from build123d import *

# Parameters (mm, degrees)
SKETCH1_R           = 7.5
BOSS_EXTRUDE1_DEPTH = 8
SKETCH2_R           = 7.5
BOSS_EXTRUDE2_DEPTH = 2
SKETCH3_R           = 4
BOSS_EXTRUDE3_DEPTH = 20
SKETCH4_R           = 5
BOSS_EXTRUDE4_DEPTH = 15


with BuildPart() as part:
    # Sketch1 → Boss-Extrude1 (new body)
    with BuildSketch(Plane(origin=(0, 0, 0), x_dir=(1, 0, 0), z_dir=(0, 1, 0))):
        Circle(SKETCH1_R)
        Polygon((5.773502692, 0), (2.886751346, 5), (-2.886751346, 5), (-5.773502692, 0), (-2.886751346, -5), (2.886751346, -5), align=None, mode=Mode.SUBTRACT)
    extrude(amount=BOSS_EXTRUDE1_DEPTH)

    # Sketch2 → Boss-Extrude2 (add)
    with BuildSketch(Plane.XZ):
        Circle(SKETCH2_R)
    extrude(amount=BOSS_EXTRUDE2_DEPTH)

    # Sketch3 → Boss-Extrude3 (add)
    with BuildSketch(Plane.XZ.offset(2)):
        Circle(SKETCH3_R)
    extrude(amount=BOSS_EXTRUDE3_DEPTH)

    # Sketch4 → Boss-Extrude4 (add)
    with BuildSketch(Plane.XZ.offset(22)):
        Circle(SKETCH4_R)
    extrude(amount=BOSS_EXTRUDE4_DEPTH)


solid = part.part
The model under review builds one solid part; all positions refer to its coordinate system, in mm. A direction names the side the tool comes from. Give positions to 0.01 mm unless a question says otherwise; leave off trailing zeros. Loops run counter-clockwise (first coordinate to the right, second up) from the corner with the lowest first, then second, coordinate; pieces in that order, holes last. Notation, with made-up numbers: (39.5, 6.25) -> (46.5, 6.25) arc R5 ccw to (46.5, 12.25) -> close; hole circle Ø10 at (41, 84.5). An arc over 180 degrees is marked (long way). Put each result on its own line as item: value. Start each with the question number.
1. We need section B-B on x = 4.5. State the section outline as (y, z) points, then the cut area to 3 significant figures.
2. We need section A-A on x = 0. State the section outline as (y, z) points, then the cut area to 3 significant figures.
3. We need section D-D on y = -24. State the section outline as (x, z) points.
4. For faces 4 (the face through (-7.493, 3.07, 0.33)), 5 (the face through (-0.867, -11.86, -3.905)), 6 (the face through (4.35, 3.944, -2.465)), list the 3-axis set-ups (+Z, -Z, +X, -X, +Y, -Y) from which the entire face can be reached by the end or side of a thin tool; tool diameter is ignored.
5. Mouldability with a two-part tool opening along X and no side actions: class faces 1 (the face through (-4.31, 3.944, -2.535)), 2 (the face through (5, 8, -2)), 3 (the face through (-1.08, -29.4, -4.88)) as released by +X, released by -X, zero draft, split by the parting line, or undercut.
6. Wall thickness on probe 1 along Y at (x, z) = (-2.75, -2.5); probe 2 along Y at (x, z) = (2.75, -4.5); probe 3 along Y at (x, z) = (-0.75, -4.75): over which ranges is each line inside the solid? List them lowest first.
7. We need section C-C on z = 2. State the section outline as (x, y) points.
8. Clearance check with flat-ended pins moving along their axes: P1, Ø4, axis at y = 1, z = 4, coming from the -X side; P2, Ø1, axis at x = 2.5, y = -14.5, coming from the +Z side; P3, Ø3, axis at x = -0.5, z = -1, coming from the +Y side. State where each tip first meets the part, or that it passes through.
Determined:
1. outline: (-37, -2.18) -> (-22, -2.18) -> (-22, 2.18) -> (-37, 2.18) -> close; (-2, -6) -> (8, -6) -> (8, -2.21) -> (0, -2.21) -> (0, 2.21) -> (8, 2.21) -> (8, 6) -> (-2, 6) -> close
1. area: 150 mm^2
2. outline: (-37, -5) -> (-22, -5) -> (-22, -4) -> (-2, -4) -> (-2, -7.5) -> (8, -7.5) -> (8, -5) -> (0, -5) -> (0, 5) -> (8, 5) -> (8, 7.5) -> (-2, 7.5) -> (-2, 4) -> (-22, 4) -> (-22, 5) -> (-37, 5) -> close
2. area: 380 mm^2
3. outline: circle Ø10 at (0, 0)
4. face 4: +Y, -Y
4. face 5: none
4. face 6: +Y
5. face 1: undercut
5. face 2: zero draft
5. face 3: split by the parting line
6. probe 1: -37 to 0
6. probe 2: -2 to 0
6. probe 3: -37 to -22, -2 to 0
7. outline: (-7.23, -2) -> (-3.46, -2) -> (-3.46, -22) -> (-4.58, -22) -> (-4.58, -37) -> (4.58, -37) -> (4.58, -22) -> (3.46, -22) -> (3.46, -2) -> (7.23, -2) -> (7.23, 8) -> (4.62, 8) -> (4.62, 0) -> (-4.62, 0) -> (-4.62, 8) -> (-7.23, 8) -> close
8. P1: x = -7.23
8. P2: z = 3.46
8. P3: y = 0
